from build123d import *

# Parameters (mm, degrees)
SKETCH3_W           = 7.62
SKETCH3_H           = 7.62
BOSS_EXTRUDE2_DEPTH = 6.35
SKETCH6_R           = 1.35255
CUT_EXTRUDE1_DEPTH  = 3.81
SKETCH7_R           = 1.35255
CUT_EXTRUDE2_DEPTH  = 2.54


with BuildPart() as part:
    # Sketch3 → Boss-Extrude2 (new body)
    with BuildSketch(Plane.XY):
        with BuildLine():
            Line((-5.207, 2.786051193), (-5.207, -6.35))
            ThreePointArc((-5.207, -6.35), (0, -8.992049984), (5.207, -6.35))
            Line((5.207, -6.35), (5.207, 2.786051193))
            ThreePointArc((5.207, 2.786051193), (0, 5.9055), (-5.207, 2.786051193))
        make_face()
        with Locations((0, -2.54)):
            Rectangle(SKETCH3_W, SKETCH3_H, mode=Mode.SUBTRACT)
    extrude(amount=BOSS_EXTRUDE2_DEPTH)

    # Sketch6 → Cut-Extrude1 (cut)
    with BuildSketch(Plane(origin=(0, 5.9055, 0), x_dir=(1, 0, 0), z_dir=(0, 1, 0))):
        with Locations(Location((0, -3.214346547, 0), (0, 0, 180))):
            Circle(SKETCH6_R)
    extrude(amount=-CUT_EXTRUDE1_DEPTH, mode=Mode.SUBTRACT)

    # Sketch7 → Cut-Extrude2 (cut)
    with BuildSketch(Plane(origin=(0, -8.992049984, 0), x_dir=(-1, 0, 0), z_dir=(0, -1, 0))):
        with Locations(Location((0, -3.175, 0), (0, 0, 180))):
            Circle(SKETCH7_R)
    extrude(amount=-CUT_EXTRUDE2_DEPTH, mode=Mode.SUBTRACT)


solid = part.part
Design review of the part built by this model. Coordinates are the model's own, in mm. A direction names the side the tool comes from. Round coordinates to 2 decimals unless told otherwise and drop trailing zeros. Loops run counter-clockwise (first coordinate to the right, second up) from the corner with the lowest first, then second, coordinate; pieces in that order, holes last. Notation, with made-up numbers: (8.5, -28.5) -> (23.5, -28.5) arc R22 ccw to (23.5, -7.5) -> close; hole circle Ø9 at (70, -20). An arc over 180 degrees is marked (long way). Use one line per item in the form item = value. Start each with the question number.
Q1. Draft analysis for pull direction Y (two halves, no side actions). For faces 1 (the face through (1.49, 5.715, 2.425)), 2 (the face through (-0.293, -7.74, 1.855)), 3 (the face through (3.81, -3, 3)), 4 (the face through (0, 1.27, 3)), state which applies: +Y half, -Y half, draft (parallel to the pull), parting line (faces both ways), or undercut.
Q2. Machinability: for faces 5 (the face through (0.176, 4.027, 4.555)), 6 (the face through (-1.42, -8.834, 3.836)), 7 (the face through (-3.81, -3, 3)), which of the approach directions +Z, -Z, +X, -X, +Y, -Y give a long, thin tool a straight path to every point of the face, cutting with its end or side? Answer none if there is none.
Q3. Wall thickness on line 1 along X through (y, z) = (-4.5, 5); line 2 along Z through (x, y) = (0, -7.6); line 3 along Z through (x, y) = (0, 3.45): over which ranges is each line inside the solid? List them lowest first. Write a range as [from, to].
Q4. For pin 1 Ø0.8 at (x, z) = (0.5, 2.5) entering from -Y; pin 2 Ø1.6 at (x, z) = (0, 3.175) entering from +Y, all flat-tipped, find the tip position at first contact; note any pin that passes through.
Q5. We need section C-C on x = 0. Give the boundary of the cut face in (y, z).
Q6. We need section D-D on y = 4. Give the boundary of the cut face in (x, z).
Q7. We need section B-B on y = -5.25. Give the boundary of the cut face in (x, z).
Q8. We need section A-A on z = 0.5. Give the boundary of the cut face in (x, y), then the cut area to 3 significant figures.
Calculated:
q1.face_1 = +Y half
q1.face_2 = draft
q1.face_3 = undercut
q1.face_4 = undercut
q2.face_5 = +Y
q2.face_6 = +Z, -Z, -Y
q2.face_7 = +Z, -Z
q3.line_1 = [-5.21, -3.81], [3.81, 5.21]
q3.line_2 = [0, 1.82], [4.53, 6.35]
q3.line_3 = [0, 1.86], [4.57, 6.35]
q4.pin_1 = -6.45
q4.pin_2 = 2.1
q5.outline = (-8.99, 0) -> (-6.35, 0) -> (-6.35, 6.35) -> (-8.99, 6.35) -> (-8.99, 4.53) -> (-6.45, 4.53) -> (-6.45, 1.82) -> (-8.99, 1.82) -> close; (1.27, 0) -> (5.91, 0) -> (5.91, 1.86) -> (2.1, 1.86) -> (2.1, 4.57) -> (5.91, 4.57) -> (5.91, 6.35) -> (1.27, 6.35) -> close
q6.outline = (-4.34, 0) -> (4.34, 0) -> (4.34, 6.35) -> (-4.34, 6.35) -> close; hole circle Ø2.71 at (0, 3.21)
q7.outline = (-5.21, 0) -> (-3.81, 0) -> (-3.81, 6.35) -> (-5.21, 6.35) -> close; (3.81, 0) -> (5.21, 0) -> (5.21, 6.35) -> (3.81, 6.35) -> close
q8.outline = (-5.21, -6.35) arc R6.45 ccw to (5.21, -6.35) -> (5.21, 2.79) arc R5.91 ccw to (-5.21, 2.79) -> close; hole (-3.81, -6.35) -> (3.81, -6.35) -> (3.81, 1.27) -> (-3.81, 1.27) -> close
q8.area = 79.5 mm²
